Read the model definition and answer for the solid it produces. Units are mm, in the model's axes. Face numbers are marked on the shaded views. A direction names the side the tool comes from. Coordinates: 2 decimals unless noted, no trailing zeros. Order: outer loops, then holes, each group sorted by start corner. A loop starts at its lowest first (then second) coordinate and runs counter-clockwise, first axis right, second up. Notation, with made-up numbers: M 89.25,-26 L 103.25,-26 A19 cw 103.25,10 Z; hole C 32.5,-16.5 d1. An arc over 180 degrees is marked long. Put each result on its own line as item: value.
from build123d import *

# Parameters (mm, degrees)
BOSS_EXTRUDE1_DEPTH = 52
CUT_EXTRUDE1_DEPTH  = 52
CHAMFER2_SIZE       = 10
SKETCH3_W           = 8
SKETCH3_H           = 4
CUT_EXTRUDE2_DEPTH  = 52
FILLET1_R           = 25
SKETCH4_W           = 3
SKETCH4_H           = 5
CUT_EXTRUDE3_DEPTH  = 52
BOSS_EXTRUDE2_DEPTH = 2
SKETCH6_R           = 2
CUT_EXTRUDE4_DEPTH  = 21


with BuildPart() as part:
    # Sketch1 → Boss-Extrude1 (new body)
    with BuildSketch(Plane(origin=(0, 0, 0), x_dir=(1, 0, 0), z_dir=(0, 1, 0))):
        Polygon((-41, -7.5), (-30, -7.5), (-30, -2.5), (30, -2.5), (30, -7.5), (41, -7.5), (41, 7.5), (-41, 7.5), align=None)
    extrude(amount=BOSS_EXTRUDE1_DEPTH)

    # Sketch2 → Cut-Extrude1 (cut)
    with BuildSketch(Plane(origin=(0, 52, 0), x_dir=(1, 0, 0), z_dir=(0, 1, 0))):
        Polygon((-41, -4.5), (-33, -4.5), (-33, 0.5), (33, 0.5), (33, -4.5), (41, -4.5), (41, 7.5), (33, 7.5), (-33, 7.5), (-41, 7.5), align=None)
    extrude(amount=-CUT_EXTRUDE1_DEPTH, mode=Mode.SUBTRACT)

    # Chamfer2
    # the kernel refuses this chamfer: 10 mm, written as the material it adds along each edge
    with BuildSketch(Plane(origin=(30, 0, 2.5), x_dir=(-0.9996219169112968, 0, -0.02749587661058636), z_dir=(0, 1, 0))) as chamfer2_piece_1_section:
        Polygon((CHAMFER2_SIZE * 0.999621916911, CHAMFER2_SIZE * 0.0274958766106), (-CHAMFER2_SIZE * 0.0274958766106, CHAMFER2_SIZE * 0.999621916911), (0, 0), align=None)
    chamfer2_piece_1 = extrude(amount=52, mode=Mode.PRIVATE)
    chamfer2_piece_1 = split(chamfer2_piece_1, bisect_by=Plane(origin=(26.065989159, 26, 7.5), z_dir=(0, 0, -1)), keep=Keep.TOP, mode=Mode.PRIVATE)
    add(chamfer2_piece_1)
    with BuildSketch(Plane(origin=(-30, 0, 2.5), x_dir=(-0.027495876610586317, 0, 0.9996219169112968), z_dir=(0, 1, 0))) as chamfer2_piece_2_section:
        Polygon((CHAMFER2_SIZE * 0.999621916911, CHAMFER2_SIZE * 0.0274958766106), (-CHAMFER2_SIZE * 0.0274958766106, CHAMFER2_SIZE * 0.999621916911), (0, 0), align=None)
    chamfer2_piece_2 = extrude(amount=52, mode=Mode.PRIVATE)
    chamfer2_piece_2 = split(chamfer2_piece_2, bisect_by=Plane(origin=(-26.065989159, 26, 7.5), z_dir=(0, 0, -1)), keep=Keep.TOP, mode=Mode.PRIVATE)
    add(chamfer2_piece_2)

    # Sketch3 → Cut-Extrude2 (cut)
    with BuildSketch(Plane.XY.offset(2.5)):
        with Locations((0, 9)):
            Rectangle(SKETCH3_W, SKETCH3_H)
    extrude(amount=-CUT_EXTRUDE2_DEPTH, mode=Mode.SUBTRACT)

    # Fillet1
    # the kernel refuses this fillet: 25 mm, written as the material it takes off along each edge
    with BuildSketch(Plane(origin=(25, -25, 7.5), x_dir=(-0.7071067811862641, 0, -0.7071067811868309), z_dir=(0, 1, 0)), Plane(origin=(-25, 77, 7.5), x_dir=(0.7071067811868301, 0, -0.7071067811862649), z_dir=(0, -1, 0))) as fillet1_piece_1:
        with BuildLine():
            CenterArc((10.606601718, -24.748737342), FILLET1_R, 98.130102354, 36.869897646)
            Line((-7.071067812, -7.071067812), (-7.424621202, -6.717514421))
            Line((-7.424621202, -6.717514421), (-0.353553391, 0.353553391))
            Line((-0.353553391, 0.353553391), (0, 0.5))
            ThreePointArc((0, 0.5), (3.535533906, 0.5), (7.000357134, 0.494974747))
            Line((7.000357134, 0.494974747), (7.071067812, 0))
        make_face()
    extrude(amount=102, mode=Mode.SUBTRACT)

    # Sketch4 → Cut-Extrude3 (cut)
    with BuildSketch(Plane(origin=(0, 52, 0), x_dir=(1, 0, 0), z_dir=(0, 1, 0))):
        with Locations((-31.5, -2)):
            Rectangle(SKETCH4_W, SKETCH4_H)
        with Locations((31.5, -2)):
            Rectangle(SKETCH4_W, SKETCH4_H)
    extrude(amount=-CUT_EXTRUDE3_DEPTH, mode=Mode.SUBTRACT)

    # Sketch5 → Boss-Extrude2 (add)
    with BuildSketch(Plane(origin=(0, 52, 0), x_dir=(1, 0, 0), z_dir=(0, 1, 0))):
        Polygon((-30, 0.5), (30, 0.5), (30, -4.5), (41, -4.5), (41, 7.5), (30, 7.5), (-30, 7.5), (-41, 7.5), (-41, -4.5), (-30, -4.5), align=None)
    extrude(amount=-BOSS_EXTRUDE2_DEPTH)

    # Sketch6 → Cut-Extrude4 (cut)
    with BuildSketch(Plane(origin=(0, 52, 0), x_dir=(1, 0, 0), z_dir=(0, 1, 0))):
        with Locations(Location((-25, 3.96, 0), (0, 0, 270))):
            Circle(SKETCH6_R)
        with Locations(Location((-10, 3.96, 0), (0, 0, 270))):
            Circle(SKETCH6_R)
        with Locations(Location((5, 3.96, 0), (0, 0, 270))):
            Circle(SKETCH6_R)
        with Locations(Location((25, 3.96, 0), (0, 0, 270))):
            Circle(SKETCH6_R)
    extrude(amount=-CUT_EXTRUDE4_DEPTH, mode=Mode.SUBTRACT)


solid = part.part
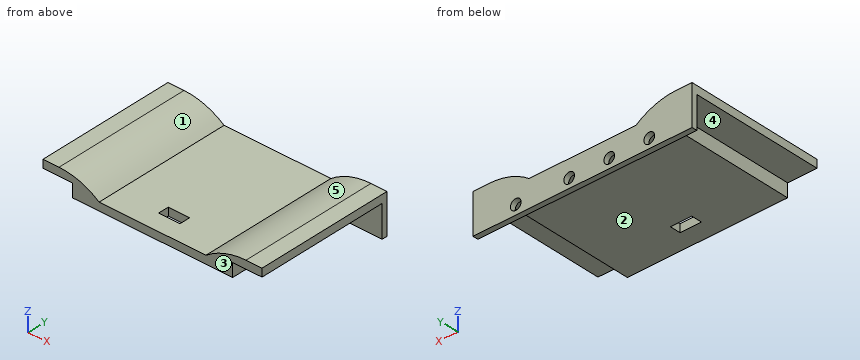
Q1. For a pull along X with two mould halves and no side action, classify the marked faces 4 and 5 as +X half, -X half, draft (parallel to the pull), parting line (faces both ways), or undercut.
Answers below:
face 4: draft
face 5: undercut
Q2. Find section D-D on y = 28. Write down the section's boundary in (x, z), plus the area to 3 significant figures.
Answers below:
outline: M -41,4.5 L -30,4.5 L -30,-0.5 L 30,-0.5 L 30,4.5 L 41,4.5 L 41,7.5 L 35,7.5 A25 ccw 20,2.5 L -20,2.5 A25 ccw -35,7.5 L -41,7.5 Z
area: 298 mm^2
Q3. Given pin 1 (2.5 mm diameter, centred on x = 1, z = 1.5, fed in from -Y); pin 2 (2.5 mm diameter, centred on y = 9.5, z = 1, fed in from +X); pin 3 (6 mm diameter, centred on x = 14, y = 32.5, fed in from -Z); pin 4 (5.5 mm diameter, centred on x = -34.5, y = 32, fed in from -Z), each flat-ended and moving along its own axis, determine where each tip first touches the part or whether it passes through.
Answers below:
pin 1: stops at y = 0
pin 2: stops at x = 30
pin 3: stops at z = -0.5
pin 4: stops at z = 4.5
Q4. A tool of negligible diameter and unlimited length cuts with its end or side. For the marked faces 1, 2 and 3, from which of +Z, -Z, +X, -X, +Y, -Y can it reach the whole face along a straight path? Write none if from no direction.
Answers below:
face 1: +Z, +Y, -Y
face 2: -Z, +X, -X, -Y
face 3: +Z, -Z, +X, -X, -Y
Q5. Consider line 1 along X through (y, z) = (51.4, -3.96); line 2 along Y through (x, z) = (0.5, 1); line 3 along Y through (x, z) = (7, -3). Determine where each line is inside the solid, lowest interval first.
Answers below:
line 1: x = -41 to -27, -23 to -12, -8 to 3, 7 to 23, 27 to 41
line 2: y = 0 to 7, 11 to 52
line 3: y = 50 to 52
Q6. Find section A-A on x = -10. Write down the section's boundary in (y, z).
Answers below:
outline: M 0,-0.5 L 50,-0.5 L 50,-1.96 L 52,-1.96 L 52,2.5 L 0,2.5 Z; M 50,-7.5 L 52,-7.5 L 52,-5.96 L 50,-5.96 Z
Q7. Find section B-B on z = 0.5. Write down the section's boundary in (x, y), plus the area to 3 significant figures.
Answers below:
outline: M -41,50 L -30,50 L -30,0 L 30,0 L 30,50 L 41,50 L 41,52 L -41,52 Z; hole M -4,7 L 4,7 L 4,11 L -4,11 Z
area: 3,130 mm^2
Q8. Find section C-C on z = -3.96. Write down the section's boundary in (x, y).
Answers below:
outline: M -41,50 L -27,50 L -27,52 L -41,52 Z; M -23,50 L -12,50 L -12,52 L -23,52 Z; M -8,50 L 3,50 L 3,52 L -8,52 Z; M 7,50 L 23,50 L 23,52 L 7,52 Z; M 27,50 L 41,50 L 41,52 L 27,52 Z
